Input: part model. Units: mm. Frame: model coordinates. A direction names the side the tool comes from. Coordinates: 2 decimals unless noted, no trailing zeros. Loops run counter-clockwise (first coordinate to the right, second up) from the corner with the lowest first, then second, coordinate; pieces in that order, holes last. Notation, with made-up numbers: M 45,25.25 L 62,25.25 A20 cw 62,43.25 Z; hole C 22.5,51.5 d3. An arc over 180 degrees is marked long. Use a Markdown table: item, result. Add a question column.
1. Pin query (flat end, axial travel): pin 1 (2 mm diameter, centred on x = 110.5, y = 7.5, fed in from -Z); pin 2 (3 mm diameter, centred on x = 110, z = 9.5, fed in from -Y). Return the tip coordinate at first contact, or that it passes through.
2. Line query: L1, parallel to Y at x = 110.1, z = 0; L2, parallel to Y at x = 111.1, z = -3.5; L3, parallel to Z at x = 111.95, y = 113.2. Output: solid intervals per line, ascending. Write a range as [from, to].
3. Set-up query: faces 5 (the cylindrical face through (110.665, -95.894, 0.4)), 6 (the cylindrical face through (110.665, 109.505, 1.532)). Return all of +Z, -Z, +X, -X, +Y, -Y with unobstructed straight access to the full face (end or side cutting, diameter ignored); none if empty.
4. Section C-C on y = 59.5. Output: boundary loops of the cut face in (x, z).
5. Section B-B on x = 109.9. Output: boundary loops of the cut face in (y, z), then the cut area to 3 significant figures.
6. Draft query along Y for faces 1 (the cylindrical face through (110.67, -116.66, -7.03)), 2 (the flat face through (110.665, -11.419, 8.735)), 3 (the flat face through (110.665, -11.394, 19.432)), 4 (the flat face through (108.2, 3, 14)). Return one class per face: +Y half, -Y half, draft (parallel to the pull), parting line (faces both ways), or undercut.
7. Section A-A on y = 113.2. Output: boundary loops of the cut face in (x, z), then the cut area to 3 significant figures.
```python
from build123d import *

# Parameters (mm, degrees)
SKETCH1_R             = 4
SKETCH1_R_2           = 3.999999999
BOSS_EXTRUDE1_DEPTH   = 5
BODY_MOVE_COPY1_ANGLE = 90


with BuildPart() as part:
    # Sketch1 → Boss-Extrude1 (new body)
    with BuildSketch(Plane(origin=(0, 0, 0), x_dir=(1, 0, 0), z_dir=(0, 1, 0))):
        with BuildLine():
            Line((-5.5, -9.526279442), (23.673254908, -26.369466016))
            ThreePointArc((23.673254908, -26.369466016), (26.504938869, -27.471302202), (29.53681211, -27.671855651))
            Line((29.53681211, -27.671855651), (222.349912922, -10.958908038))
            ThreePointArc((222.349912922, -10.958908038), (229.638892539, 7.288391438), (210.63878065, 2.279508305))
            ThreePointArc((210.63878065, 2.279508305), (209.060222507, -0.429302712), (206.17909591, -1.665673394))
            Line((206.17909591, -1.665673394), (40.742030274, -16.005679335))
            ThreePointArc((40.742030274, -16.005679335), (33.162347172, -15.504295714), (26.08313727, -12.749705247))
            Line((26.08313727, -12.749705247), (13.459935794, -5.461696477))
            ThreePointArc((13.459935794, -5.461696477), (11.544061041, -3.476788033), (10.972455859, -0.777954003))
            ThreePointArc((10.972455859, -0.777954003), (-5.159480863, 9.714924458), (-5.5, -9.526279442))
        make_face()
        Circle(SKETCH1_R, mode=Mode.SUBTRACT)
        with Locations((221.4, 2e-09)):
            Circle(SKETCH1_R_2, mode=Mode.SUBTRACT)
    extrude(amount=BOSS_EXTRUDE1_DEPTH)


with BuildPart() as part_1:
    # Body-Move/Copy1: moved
    add(part.part.rotate(Axis((110.7, 2.5, 0), (0, 0, -1)), BODY_MOVE_COPY1_ANGLE))


solid = part_1.part
```
Answers below:
| question | item | result |
|---|---|---|
| 1 | pin 1 | stops at z = 10.29 |
| 1 | pin 2 | stops at y = -115.75 |
| 2 | L1 | y = [-119.2, -112.2], [-104.2, -96.29], [102.2, 109.2], [117.2, 124.2] |
| 2 | L2 | y = [-118.63, -110.14], [-106.26, -97.77], [102.77, 111.26], [115.14, 123.63] |
| 2 | L3 | z = [-11, -4], [4, 12.7] |
| 3 | face 5 | -Z, +X, -X |
| 3 | face 6 | +X, -X |
| 4 | outline | M 108.2,14.88 L 113.2,14.88 L 113.2,25.58 L 108.2,25.58 Z |
| 5 | outline | M -109.15,10.96 A11 ccw long -97.44,-2.28 A5 cw -92.98,1.67 L 72.46,16.01 A25 cw 87.12,12.75 L 99.74,5.46 A5 cw 102.23,0.78 A11 ccw long 118.7,9.53 L 89.53,26.37 A10 ccw 83.66,27.67 Z; hole C -108.2,0 d8; hole C 113.2,0 d8 |
| 5 | area | 3,000 mm² |
| 6 | face 1 | undercut |
| 6 | face 2 | undercut |
| 6 | face 3 | -Y half |
| 6 | face 4 | draft |
| 7 | outline | M 108.2,-11 L 113.2,-11 L 113.2,-4 L 108.2,-4 Z; M 108.2,4 L 113.2,4 L 113.2,12.7 L 108.2,12.7 Z |
| 7 | area | 78.5 mm² |
